Here's how the part is built. I have some questions about the finished solid (model axes, mm). A direction names the side the tool comes from. Coordinates: 2 decimals unless noted, no trailing zeros. Write each loop counter-clockwise with the first axis right and the second up, starting at its lowest first coordinate (ties: lowest second). Pieces come first, ordered by that corner, then holes. Notation, with made-up numbers: (-11.75, -31) -> (11.25, -31) arc R21 cw to (11.25, -17) -> close; hole circle Ø11 at (-1.75, 32). An arc over 180 degrees is marked (long way). Use CSV: the item, a comma, the result in double quotes. Start each with the question number.
Autodesk Inventor part; units mm, degrees
ref_plane "YZ Plane" through (0, 0, 0) normal (1, 0, 0) x (0, 1, 0)
ref_plane "XZ Plane" through (0, 0, 0) normal (0, 1, 0) x (-1, 0, 0)
ref_plane "XY Plane" through (0, 0, 0) normal (0, 0, 1) x (1, 0, 0)
sketch "Skizze1" plane through (0, 0, 0) normal (0, 0, 1) x (1, 0, 0)
  line L0 (-20.1131, -4) -> (51.8869, -4)
  line L1 (51.8869, -4) -> (51.8869, 40)
  line L2 (51.8869, 40) -> (-20.1131, 40)
  line L3 (-20.1131, 40) -> (-20.1131, -4)
  arc A0 (51.8869, 40) -> (-20.1131, 40) centre (15.8869, 5.3013) ccw
  line L4 (50.3869, -4) -> (50.3869, 40)
  line L5 (-18.6131, 40) -> (-18.6131, -4)
  arc A1 (50.3869, 40) -> (-18.6131, 40) centre (15.8869, 5.2581) ccw
  point P0 (0, 0)
  dimension "d0" = 72
  dimension "d1" = 44
  dimension "d2" = 50
  dimension "d3" = 1.5
  dimension "d4" = 1.5
extrude "Extrusion1" add sketch "Skizze1" along normal blind 2 contours L5 L2 L4 L0 | A1 L2
extrude "Extrusion2" add sketch "Skizze1" along normal blind 15 contours L3 L2 L5 L0 | A0 L2 A1 | L4 L2 L1 L0
sketch "Skizze2" plane through (0, 0, 2) normal (0, 0, 1) x (1, 0, 0)
  circle A0 centre (-14.6131, 19.5) radius 3
  circle A1 centre (-14.6131, 19.5) radius 2
  circle A2 centre (45.3869, 19) radius 3
  circle A3 centre (45.3869, 19) radius 2
  line L0 (50.3869, 40) -> (50.3869, -4)
  line L1 (-18.6131, -4) -> (-18.6131, 40)
  circle A4 centre (-3.6131, 40) radius 2
  circle A5 centre (35.3869, 40) radius 2
  circle A6 centre (35.3869, 40) radius 1.05
  circle A7 centre (-3.6131, 40) radius 1.05
  line L2 (-6.6131, 32) -> (38.3869, 32)
  line L3 (38.3869, 32) -> (38.3869, 26)
  line L4 (38.3869, 26) -> (-6.6131, 26)
  line L5 (-6.6131, 26) -> (-6.6131, 32)
  line L6 (50.3869, -4) -> (43.3869, -4)
  line L7 (-18.6131, 0) -> (-13.6131, 0)
  line L8 (-13.6131, 0) -> (-13.6131, -2)
  line L9 (-13.6131, -2) -> (-18.6131, -2)
  line L10 (-18.6131, -2) -> (-18.6131, 0)
  line L11 (45.3869, 0) -> (50.3869, 0)
  line L12 (50.3869, 0) -> (50.3869, -2)
  line L13 (50.3869, -2) -> (45.3869, -2)
  line L14 (45.3869, -2) -> (45.3869, 0)
  line L15 (-18.6131, -4) -> (50.3869, -4)
  point P0 (0, 0)
  point P1 (15.8869, 26)
  point P2 (15.8869, 32)
  point P3 (-6.6131, 29)
  point P4 (38.3869, 29)
  point P5 (45.3869, -1)
  point P6 (-13.6131, -1)
  dimension "d9" = 6
  dimension "d10" = 4
  dimension "d11" = 6
  dimension "d12" = 4
  dimension "d13" = 5
  dimension "d14" = 4
  dimension "d21" = 4
  dimension "d22" = 4
  dimension "d23" = 2.1
  dimension "d24" = 2.1
  dimension "d27" = 15
  dimension "d28" = 15
  dimension "d29" = 60
  dimension "d30" = 6
  dimension "d31" = 45
  dimension "d32" = 12
  dimension "d33" = 12
  dimension "d40" = 5
  dimension "d41" = 2
  dimension "d43" = 5
  dimension "d44" = 2
  dimension "d45" = 2
  dimension "d46" = 59
  dimension "d47" = 23.5
  dimension "d48" = 23
  dimension "d49" = 44
  dimension "d50" = 44
  dimension "d51" = 30
extrude "Extrusion3" add sketch "Skizze2" along normal blind 2 contours A0 | A2 | L2 L3 L4 L5
extrude "Extrusion4" add sketch "Skizze2" along normal blind 7 contours A1 | A3
extrude "Extrusion5" add sketch "Skizze2" along normal blind 11 contours A4 | A5
extrude "Extrusion6" add sketch "Skizze2" along normal up to surface (13 mm away) contours L1 L7 L8 L9 | L0 L13 L14 L11
properties part number "Spiel"
Item 1: If I drill on line 1 along Y through (x, z) = (-3.5, 3.5); line 2 along X through (y, z) = (2, 5.25); line 3 along Z through (x, y) = (10.5, 25.5), over which ranges is the centre line in solid material (lowest first)?
Item 2: I want a section at A-A on z = 11.75. Please give me the cut outline in (x, y), then the cut area to 3 significant figures.
Item 3: I want a section at D-D on x = 19. Please give me the cut outline in (y, z).
Item 4: I want a section at C-C on y = 27. Please give me the cut outline in (x, z).
Item 5: Which directions (+Z, -Z, +X, -X, +Y, -Y) give clear straight access to the entire face, cutting with the end or side of a thin tool? Please do faces 5 (the flat face through (16, 29, 4)), 6 (the flat face through (-20.113, 18, 7)), 7 (the flat face through (48, 0, 8)).
Item 6: Thinking about a two-plate mould opening in Y: for faces 1 (the flat face through (16, 32, 3)), 2 (the cylindrical face through (34.34, 39.95, 7.42)), 3 (the flat face through (48, -2, 8)), 4 (the flat face through (45.387, -1, 8)), which applies, +Y half, -Y half, draft (parallel to the pull), parting line (faces both ways), or undercut?
Item 7: I'm going to push flat-ended pins straight in: pin 1 (3 mm diameter, centred on x = -15, y = 20.5, fed in from +Z); pin 2 (10 mm diameter, centred on x = 3.5, y = 24.5, fed in from +Z); pin 3 (1.2 mm diameter, centred on x = 35.5, y = 39, fed in from +Z). Where does each tip first touch, or does it pass through?
Item 8: I want a section at B-B on z = 8. Please give me the cut outline in (x, y).
Geometry says:
1,line 1,"26 to 32, 38 to 38.96, 41.04 to 42, 50.22 to 51.39"
1,line 2,"-20.11 to -18.61, 50.39 to 51.89"
1,line 3,"0 to 2"
2,outline,"(-20.11, -4) -> (-18.61, -4) -> (-18.61, -2) -> (-13.61, -2) -> (-13.61, 0) -> (-18.61, 0) -> (-18.61, 40) arc R48.96 cw to (50.39, 40) -> (50.39, 0) -> (45.39, 0) -> (45.39, -2) -> (50.39, -2) -> (50.39, -4) -> (51.89, -4) -> (51.89, 40) arc R50 ccw to (-20.11, 40) -> close; circle Ø4 at (-3.61, 40); circle Ø4 at (35.39, 40); hole circle Ø2.1 at (-3.61, 40); hole circle Ø2.1 at (35.39, 40)"
2,area,"255 mm2"
3,outline,"(-4, 0) -> (55.2, 0) -> (55.2, 15) -> (54.12, 15) -> (54.12, 2) -> (32, 2) -> (32, 4) -> (26, 4) -> (26, 2) -> (-4, 2) -> close"
4,outline,"(-20.11, 0) -> (51.89, 0) -> (51.89, 15) -> (50.39, 15) -> (50.39, 2) -> (38.39, 2) -> (38.39, 4) -> (-6.61, 4) -> (-6.61, 2) -> (-18.61, 2) -> (-18.61, 15) -> (-20.11, 15) -> close"
5,face 5,"+Z, -Y"
5,face 6,"+Z, -Z, -X, +Y, -Y"
5,face 7,"+Z"
6,face 1,"undercut"
6,face 2,"undercut"
6,face 3,"-Y half"
6,face 4,"draft"
7,pin 1,"z = 9"
7,pin 2,"z = 4"
7,pin 3,"z = 13"
8,outline,"(-20.11, -4) -> (-18.61, -4) -> (-18.61, -2) -> (-13.61, -2) -> (-13.61, 0) -> (-18.61, 0) -> (-18.61, 40) arc R48.96 cw to (50.39, 40) -> (50.39, 0) -> (45.39, 0) -> (45.39, -2) -> (50.39, -2) -> (50.39, -4) -> (51.89, -4) -> (51.89, 40) arc R50 ccw to (-20.11, 40) -> close; circle Ø4 at (-14.61, 19.5); circle Ø4 at (-3.61, 40); circle Ø4 at (35.39, 40); circle Ø4 at (45.39, 19); hole circle Ø2.1 at (-3.61, 40); hole circle Ø2.1 at (35.39, 40)"
